```python
from build123d import *

# Parameters (mm, degrees)
BOSS_EXTRUDE1_DEPTH      = 116.205
BOSS_EXTRUDE1_DEPTH_BACK = 116.205
SKETCH1_W                = 6.35
SKETCH1_H                = 6.35
SKETCH1_R                = 1.397
BOSS_EXTRUDE3_DEPTH      = 249.936
BOSS_EXTRUDE3_DEPTH_BACK = 249.936
SKETCH3_R                = 1.9939
SKETCH3_R_2              = 1.397


with BuildPart() as part:
    # Sketch1 → Boss-Extrude1 (new, two sides: drawn at the far end of the back side and taken through both)
    with BuildSketch(Plane(origin=(0, 0, 0), x_dir=(0, 0, -1), z_dir=(1, 0, 0)).offset(-BOSS_EXTRUDE1_DEPTH_BACK)):
        with Locations((3.175, 3.175)):
            Rectangle(SKETCH1_W, SKETCH1_H)
        with Locations((3.175, 3.175)):
            Circle(SKETCH1_R, mode=Mode.SUBTRACT)
    extrude(amount=BOSS_EXTRUDE1_DEPTH + BOSS_EXTRUDE1_DEPTH_BACK)

    # Sketch3 → Boss-Extrude3 (add, two sides: drawn at the far end of the back side and taken through both)
    with BuildSketch(Plane(origin=(0, 0, 0), x_dir=(0, 0, -1), z_dir=(1, 0, 0)).offset(-BOSS_EXTRUDE3_DEPTH_BACK)):
        with Locations((3.175, 3.175)):
            Circle(SKETCH3_R)
        with Locations((3.175, 3.175)):
            Circle(SKETCH3_R_2, mode=Mode.SUBTRACT)
    extrude(amount=BOSS_EXTRUDE3_DEPTH + BOSS_EXTRUDE3_DEPTH_BACK)


solid = part.part
```
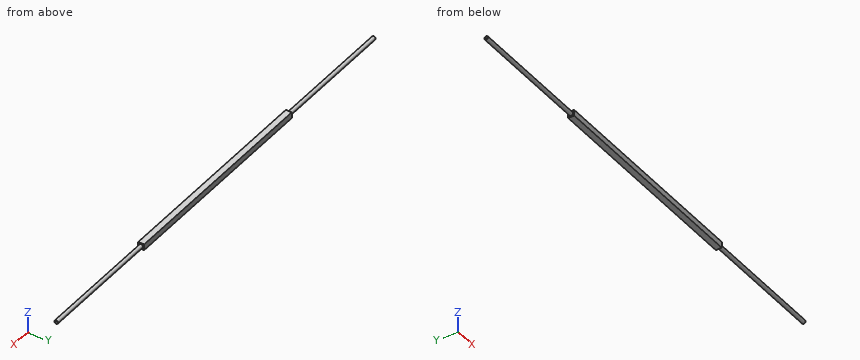
Work out the finished part from the listing and answer in its coordinate system (mm). Coordinates: 2 decimals unless noted, no trailing zeros. Write each loop counter-clockwise with the first axis right and the second up, starting at its lowest first coordinate (ties: lowest second). Pieces come first, ordered by that corner, then holes.
Q1. A cutting plane is placed at A-A, the plane x = 47. Give the vertices of the cut face in (y, z) (3 decimals), then the cut area to 3 significant figures.
Q2. Find the intervals of material crossed by line 1 (Z direction, x = 25.5, y = 3); line 2 (Z direction, x = -180.5, y = 3.5); line 3 (Y direction, x = 59, z = -3), in increasing order.
Q3. A cutting plane is placed at B-B, the plane x = -173. Give the vertices of the cut face in (y, z) (3 decimals), then the cut area to 3 significant figures.
Findings below:
1. outline: (0, -6.35) - (6.35, -6.35) - (6.35, 0) - (0, 0) - close; hole circle Ø2.794 at (3.175, -3.175)
1. area: 34.2 mm2
2. line 1: z = -6.35 to -4.56, -1.79 to 0
2. line 2: z = -5.14 to -4.53, -1.82 to -1.21
2. line 3: y = 0 to 1.79, 4.56 to 6.35
3. outline: circle Ø3.988 at (3.175, -3.175); hole circle Ø2.794 at (3.175, -3.175)
3. area: 6.36 mm2
